Autodesk Inventor part; units mm, degrees
ref_plane "YZ Plane" through (0, 0, 0) normal (1, 0, 0) x (0, 1, 0)
ref_plane "XZ Plane" through (0, 0, 0) normal (0, 1, 0) x (-1, 0, 0)
ref_plane "XY Plane" through (0, 0, 0) normal (0, 0, 1) x (1, 0, 0)
sketch "Sketch1" plane through (0, 0, 0) normal (0, 0, 1) x (1, 0, 0)
  circle A0 centre (0, 0) radius 45
  circle A1 centre (0, 0) radius 38
  line L0 (0, 0) -> (0, -38) construction
  line L1 (-1.25, -17) -> (1.25, -17)
  line L2 (1.25, -17) -> (1.05, -34)
  line L3 (1.05, -34) -> (-1.05, -34)
  line L4 (-1.25, -17) -> (-1.05, -34)
  circle A2 centre (0, 0) radius 1.5
  circle A3 centre (0, -9.53) radius 1.6035
  circle A4 centre (8.2532, -4.765) radius 1.6035
  circle A5 centre (8.2532, 4.765) radius 1.6035
  circle A6 centre (0, 9.53) radius 1.6035
  circle A7 centre (-8.2532, 4.765) radius 1.6035
  circle A8 centre (-8.2532, -4.765) radius 1.6035
  line L5 (0, -9.53) -> (8.2532, -4.765) construction
  line L6 (4.1266, -7.1475) -> (3.7658, -37.8129)
  line L7 (0, -9.53) -> (-8.2532, -4.765) construction
  line L8 (-4.1266, -7.1475) -> (-3.7658, -37.8129)
  line L9 (14.0974, -9.5825) -> (15.3474, -7.4175)
  line L10 (15.3474, -7.4175) -> (29.9699, -16.0907)
  line L11 (29.9699, -16.0907) -> (28.9199, -17.9093)
  line L12 (14.0974, -9.5825) -> (28.9199, -17.9093)
  line L13 (8.2532, 0) -> (34.6299, -15.6452)
  line L14 (4.1266, -7.1475) -> (30.864, -22.1678)
  line L15 (15.3474, 7.4175) -> (14.0974, 9.5825)
  line L16 (14.0974, 9.5825) -> (28.9199, 17.9093)
  line L17 (28.9199, 17.9093) -> (29.9699, 16.0907)
  line L18 (15.3474, 7.4175) -> (29.9699, 16.0907)
  line L19 (4.1266, 7.1475) -> (30.864, 22.1678)
  line L20 (8.2532, 0) -> (34.6299, 15.6452)
  line L21 (1.25, 17) -> (-1.25, 17)
  line L22 (-1.25, 17) -> (-1.05, 34)
  line L23 (-1.05, 34) -> (1.05, 34)
  line L24 (1.25, 17) -> (1.05, 34)
  line L25 (-4.1266, 7.1475) -> (-3.7658, 37.8129)
  line L26 (4.1266, 7.1475) -> (3.7658, 37.8129)
  line L27 (-14.0974, 9.5825) -> (-15.3474, 7.4175)
  line L28 (-15.3474, 7.4175) -> (-29.9699, 16.0907)
  line L29 (-29.9699, 16.0907) -> (-28.9199, 17.9093)
  line L30 (-14.0974, 9.5825) -> (-28.9199, 17.9093)
  line L31 (-8.2532, 0) -> (-34.6299, 15.6452)
  line L32 (-4.1266, 7.1475) -> (-30.864, 22.1678)
  line L33 (-15.3474, -7.4175) -> (-14.0974, -9.5825)
  line L34 (-14.0974, -9.5825) -> (-28.9199, -17.9093)
  line L35 (-28.9199, -17.9093) -> (-29.9699, -16.0907)
  line L36 (-15.3474, -7.4175) -> (-29.9699, -16.0907)
  line L37 (-4.1266, -7.1475) -> (-30.864, -22.1678)
  line L38 (-8.2532, 0) -> (-34.6299, -15.6452)
  line L39 (3.7658, -37.8129) -> (4.1266, -7.1475)
  line L40 (30.864, -22.1678) -> (4.1266, -7.1475)
  arc A9 (-30.864, -22.1678) -> (-3.7658, -37.8129) centre (0, 0) ccw
  arc A10 (3.7658, -37.8129) -> (30.864, -22.1678) centre (0, 0) ccw
  line L41 (-30.864, -22.1678) -> (-4.1266, -7.1475)
  line L42 (-4.1266, -7.1475) -> (-3.7658, -37.8129)
  line L43 (-34.6299, -15.6452) -> (-8.2532, 0)
  line L44 (-34.6299, 15.6452) -> (-8.2532, 0)
  line L45 (-4.1266, 7.1475) -> (-30.864, 22.1678)
  line L46 (-4.1266, 7.1475) -> (-3.7658, 37.8129)
  line L47 (4.1266, 7.1475) -> (3.7658, 37.8129)
  line L48 (4.1266, 7.1475) -> (30.864, 22.1678)
  line L49 (34.6299, 15.6452) -> (8.2532, 0)
  line L50 (8.2532, 0) -> (34.6299, -15.6452)
  arc A11 (-34.6299, 15.6452) -> (-34.6299, -15.6452) centre (0, 0) ccw
  arc A12 (-3.7658, 37.8129) -> (-30.864, 22.1678) centre (0, 0) ccw
  arc A13 (30.864, 22.1678) -> (3.7658, 37.8129) centre (0, 0) ccw
  arc A14 (34.6299, -15.6452) -> (34.6299, 15.6452) centre (0, 0) ccw
  arc A15 (-3.7658, 37.8129) -> (-30.864, 22.1678) centre (0, 0) ccw
  arc A16 (-3.7658, 37.8129) -> (-30.864, 22.1678) centre (0, 0) ccw
  line L51 (-30.864, 22.1678) -> (-4.1266, 7.1475)
  line L52 (-4.1266, 7.1475) -> (-3.7658, 37.8129)
  point P0 (32.909, -19)
  point P1 (8.2532, -4.765)
  point P2 (32.909, 19)
  point P3 (8.2532, 4.765)
  point P4 (0, 38)
  point P5 (0, 9.53)
  point P6 (-32.909, 19)
  point P7 (-8.2532, 4.765)
  point P8 (-32.909, -19)
  point P9 (-8.2532, -4.765)
  dimension "d0" = 90
  dimension "d1" = 76
  dimension "d2" = 2.1
  dimension "d3" = 2.5
  dimension "d4" = 1.25
  dimension "d5" = 1.05
  dimension "d6" = 3
  dimension "d7" = 17
  dimension "d8" = 4
  dimension "d9" = 9.53
  dimension "d12" = 360
  dimension "d16" = 360
  dimension "d20" = 3.207
extrude "Extrusion1" add sketch "Sketch1" along normal mid plane 10 contours A0
extrude "Extrusion2" add sketch "Sketch1" along normal mid plane 4 contours L20 L13 A1 L14 L6 L8 L37 L38 L31 L32 L25 L26 L19
sketch "Sketch2" plane through (0, 0, 2) normal (0, 0, 1) x (1, 0, 0)
  circle A0 centre (0, 0) radius 1.5
  circle A1 centre (0, 0) radius 3.5
  dimension "d23" = 7
extrude "Extrusion3" add sketch "Sketch2" along normal blind 3.9
sketch "Sketch3" plane through (0, 0, -2) normal (0, 0, -1) x (-1, 0, 0)
  circle A0 centre (8.2532, -4.765) radius 1.6035
  circle A1 centre (8.2532, 4.765) radius 1.6035
  circle A2 centre (0, 9.53) radius 1.6035
  circle A3 centre (-8.2532, 4.765) radius 1.6035
  circle A4 centre (-8.2532, -4.765) radius 1.6035
  circle A5 centre (0, -9.53) radius 1.6035
  circle A6 centre (0, 0) radius 1.5
  circle A7 centre (0, 0) radius 12.7
  circle A8 centre (0, 0) radius 3.5
  circle A9 centre (0, 0) radius 3
  circle A10 centre (0, 0) radius 5.5
  dimension "d26" = 6
  dimension "d27" = 11
  dimension "d28" = 25.4
extrude "Extrusion4" add sketch "Sketch3" along normal blind 4.6 contours A7
extrude "Extrusion5" add sketch "Sketch3" along normal blind 9.2 contours A8 | A10
properties part number "Wheel90mm"
Geometry: final body of the model. Coordinates: model frame, mm. A direction names the side the tool comes from. Give positions to 0.01 mm unless a question says otherwise; leave off trailing zeros. Write each loop counter-clockwise with the first axis right and the second up, starting at its lowest first coordinate (ties: lowest second). Pieces come first, ordered by that corner, then holes. Notation, with made-up numbers: M 52.5,50 L 72.5,50 A14 ccw 72.5,61 Z; hole C 51.5,-26.75 d7. An arc over 180 degrees is marked long. Answer in a Markdown table with one row per item. Add a question column.
(1) Reachability of faces 1 (the flat face through (11, 0, -2)), 2 (the flat face through (-22.556, 11.693, -0.028)), 3 (the flat face through (-2, -25, -2)) from +Z, -Z, +X, -X, +Y, -Y: full face, straight path, thin tool, end or side. Return the list, or none.
(2) First-contact query: pin 1 (4 mm diameter, centred on x = 8.25, y = -4.76, fed in from -Z); pin 2 (2 mm diameter, centred on y = -3, z = 1.5, fed in from -X); pin 3 (4 mm diameter, centred on x = 1.5, y = 21, fed in from -Z). Flat tips, straight axial feed; report the tip coordinate or a pass-through.
(3) Section A-A on y = -31.5. Return loops of the section in (x, z).
(4) Section C-C on z = -9. Return loops of the section in (x, y), and give its area (3 significant figures).
(5) Mould query, pull axis Y, two halves, no side actions, for faces 4 (the flat face through (-21.257, 7.713, -0.028)), 5 (the cylindrical face through (1.19, 5.37, -8.87)). Classes: +Y half, -Y half, draft (parallel to the pull), parting line (faces both ways), or undercut.
(6) Section D-D on x = 21.5. Return loops of the section in (y, z), and give its area (3 significant figures).
(7) Section B-B on x = -11. Return loops of the section in (y, z), and give its area (3 significant figures).
(8) Ray query, line 1 (Y direction, x = 0, z = -4.35); line 2 (Y direction, x = 0, z = 1); line 3 (Y direction, x = 0, z = -5.25). Return the intervals inside material, ascending.
Result set:
| question | item | result |
|---|---|---|
| 1 | face 1 | +Z |
| 1 | face 2 | +Z, -Z |
| 1 | face 3 | -Z |
| 2 | pin 1 | stops at z = -6.6 |
| 2 | pin 2 | stops at x = -44.96 |
| 2 | pin 3 | stops at z = -2 |
| 3 | outline | M -32.14,-5 L -21.25,-5 L -21.25,5 L -32.14,5 Z; M -3.84,-2 L -1.08,-2 L -1.08,2 L -3.84,2 Z; M 1.08,-2 L 3.84,-2 L 3.84,2 L 1.08,2 Z; M 21.25,-5 L 32.14,-5 L 32.14,5 L 21.25,5 Z |
| 4 | outline | C 0,0 d11; hole C 0,0 d6 |
| 4 | area | 66.8 mm^2 |
| 5 | face 4 | undercut |
| 5 | face 5 | parting line |
| 6 | outline | M -39.53,-5 L -31.33,-5 L -31.33,5 L -39.53,5 Z; M -16.91,-2 L -13.74,-2 L -13.74,2 L -16.91,2 Z; M -11.07,-2 L -7.86,-2 L -7.86,2 L -11.07,2 Z; M 7.86,-2 L 11.07,-2 L 11.07,2 L 7.86,2 Z; M 13.74,-2 L 16.91,-2 L 16.91,2 L 13.74,2 Z; M 31.33,-5 L 39.53,-5 L 39.53,5 L 31.33,5 Z |
| 6 | area | 215 mm^2 |
| 7 | outline | M -43.63,-5 L -36.37,-5 L -36.37,5 L -43.63,5 Z; M -11.01,-2 L -6.35,-2 L -6.35,-6.6 L 6.35,-6.6 L 6.35,-2 L 11.01,-2 L 11.01,2 L 1.63,2 L 1.63,-2 L -1.63,-2 L -1.63,2 L -11.01,2 Z; M 36.37,-5 L 43.63,-5 L 43.63,5 L 36.37,5 Z |
| 7 | area | 279 mm^2 |
| 8 | line 1 | y = -45 to -38, -12.7 to -11.13, -7.93 to -3, 3 to 7.93, 11.13 to 12.7, 38 to 45 |
| 8 | line 2 | y = -45 to -34, -17 to -11.13, -7.93 to -1.5, 1.5 to 7.93, 11.13 to 17, 34 to 45 |
| 8 | line 3 | y = -12.7 to -11.13, -7.93 to -3, 3 to 7.93, 11.13 to 12.7 |
